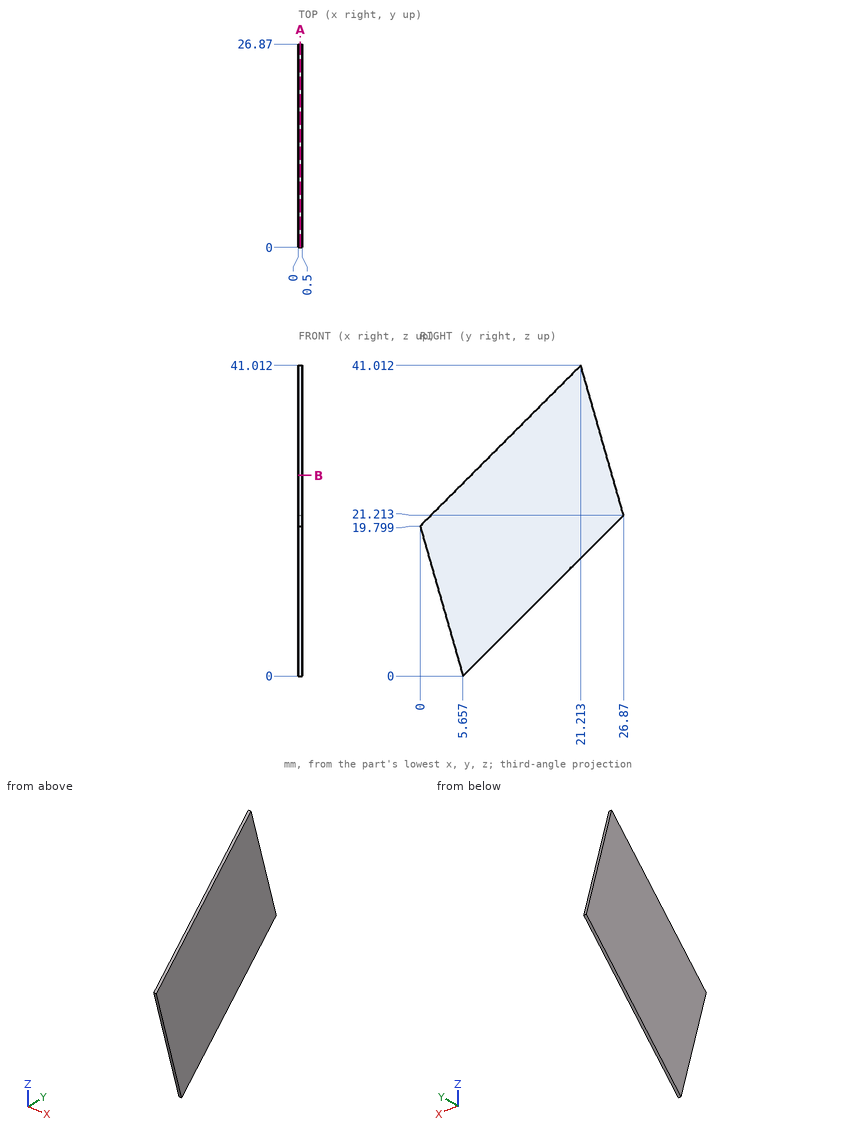
The figure shows three views and two pictorial views of one solid part (mm, origin at its lowest corner). Answer the questions. Round coordinates to 2 decimals unless told otherwise and drop trailing zeros. Write each loop counter-clockwise with the first axis right and the second up, starting at its lowest first coordinate (ties: lowest second). Pieces come first, ordered by that corner, then holes. Notation, with made-up numbers: (-23.75, 22.5) -> (1.25, 22.5) arc R11 cw to (1.25, 41.5) -> close; hole circle Ø7 at (23, -31.5). An arc over 180 degrees is marked (long way). Write each question's results on one line, items separated by ' | '.
Q1. Straight lines are drawn through the part: line 1 along Y through (x, z) = (0.1, 15.5); line 2 along Z through (x, y) = (0.3, 12); line 3 along Z through (x, y) = (0.1, 7). For each, find the intervals that lie inside material, in ascending order. Write a range as [from, to].
Data:
line 1: [1.23, 21.16] | line 2: [6.34, 31.8] | line 3: [1.34, 26.8]
Q2. Section A-A, the plane x = 0.25 is taken. Write down the section's boundary in (y, z), then the cut area to 3 significant figures.
Data:
outline: (0, 19.8) -> (5.66, 0) -> (26.87, 21.21) -> (21.21, 41.01) -> close | area: 540 mm^2
Q3. Section B-B, the plane z = 26.5 is taken. Write down the section's boundary in (x, y).
Data:
outline: (0, 6.7) -> (0.5, 6.7) -> (0.5, 25.36) -> (0, 25.36) -> close
